from build123d import *

# Parameters (mm, degrees)
F3_DEPTH = 6
F4_R     = 4.8870891215
F5_DEPTH = 4.0010006557


with BuildPart() as f1:
    # F0 (on Front) → F1 (revolve)
    with BuildSketch(Plane.XZ):
        Polygon((-7.3680463247, -9.7499769181), (-20, -9.7499769181), (-20, -13.7499775738), (0, -13.7499775738), (0, 13.7500224262), (-4, 13.4215392172), (-4, -0.5182113382), (-7.3680463247, -0.5182113382), align=None)
    revolve(axis=Axis((0, 0, 2.24262e-05), (0, 0, 1)))

    # F2 (on face) → F3 (join)
    with BuildSketch(Plane.XY.offset(-0.5182113382)):
        Polygon((-1.4578928646, 3.7248554865), (1.4578928646, 3.7248554865), (0, 6.25), align=None)
        Polygon((-3.954765909, -0.5998554865), (-5.4126587737, -3.125), (-2.4968730444, -3.125), align=None)
        Polygon((2.4968730444, -3.125), (5.4126587737, -3.125), (3.954765909, -0.5998554865), align=None)
    extrude(amount=F3_DEPTH)

    # F4 (on face) → F5 (cut, through all)
    with BuildSketch(Plane.XY.offset(-9.7499769181)):
        with Locations((12.3, 0)):
            Circle(F4_R)
    extrude(amount=-F5_DEPTH, mode=Mode.SUBTRACT)


solid = f1.part
Geometry check sheet. Reference: the model listing, model coordinates, mm. A direction names the side the tool comes from. Round coordinates to 2 decimals unless told otherwise and drop trailing zeros. Loops run counter-clockwise (first coordinate to the right, second up) from the corner with the lowest first, then second, coordinate; pieces in that order, holes last.
Item 1: Gauge pin test, flat ends, axial feed: pin 1 (0.8 mm diameter, centred on x = -0.5, y = 5.5, fed in from +Z); pin 2 (12.5 mm diameter, centred on x = 12.3, y = 0, fed in from +Z); pin 3 (2 mm diameter, centred on y = -2, z = 3, fed in from -X); pin 4 (10 mm diameter, centred on x = 15.5, z = 4, fed in from +Y). Record the tip position at first contact, or that the pin passes through.
Item 2: Access from +Z, -Z, +X, -X, +Y, -Y to the whole of each face (thin tool, end or side, straight path). Record for faces 4 (the flat face through (-0.719, 5.005, 2.44)), 5 (the cylindrical face through (-3.4, 6.537, -5.199)), 6 (the flat face through (4, -2, 5.482)).
Item 3: Cross-section at D-D on z = 11.25. Record the boundary of the cut face in (x, y).
Item 4: Cross-section at B-B on x = 12.3. Record the boundary of the cut face in (y, z).
Item 5: Thickness scan on line 1 (Z direction, x = -6, y = -14.5); line 2 (Y direction, x = 12.3, z = -11.15); line 3 (X direction, y = 4, z = -10.75). Record the ranges inside material, lowest first.
Item 6: Cross-section at C-C on y = -12. Record the boundary of the cut face in (x, z), then the cut area to 3 significant figures.
Item 7: Mould release check, pull along X, two halves, no side actions. Record for faces 1 (the cylindrical face through (0.867, 3.905, 6.354)), 2 (the flat face through (-4, -3.125, 2)), 3 (the cylindrical face through (8.42, -2.97, -11.72)): pulls with the +X half, pulls with the -X half, needs draft (parallel to the pull), parting line crosses it, or undercut.
Item 8: Cross-section at A-A on z = 2.5. Record the boundary of the cut face in (x, y) (3 decimals), then the cut area to 3 significant figures.
Answer sheet:
1. pin 1: stops at z = 5.48
1. pin 2: stops at z = -0.52
1. pin 3: stops at x = -5.34
1. pin 4: passes through
2. face 4: +Z, -X, +Y
2. face 5: +Z
2. face 6: +Z, +X, -Y
3. outline: circle Ø8 at (0, 0)
4. outline: (-15.77, -13.75) - (-4.89, -13.75) - (-4.89, -9.75) - (-15.77, -9.75) - close; (4.89, -13.75) - (15.77, -13.75) - (15.77, -9.75) - (4.89, -9.75) - close
5. line 1: z = -13.75 to -9.75
5. line 2: y = -15.77 to -4.89, 4.89 to 15.77
5. line 3: x = -19.6 to 9.49, 15.11 to 19.6
6. outline: (-16, -13.75) - (16, -13.75) - (16, -9.75) - (-16, -9.75) - close
6. area: 128 mm2
7. face 1: parting line crosses it
7. face 2: needs draft
7. face 3: undercut
8. outline: (-5.413, -3.125) - (-2.497, -3.125) arc R4 ccw to (2.497, -3.125) - (5.413, -3.125) - (3.955, -0.6) arc R4 ccw to (1.458, 3.725) - (0, 6.25) - (-1.458, 3.725) arc R4 ccw to (-3.955, -0.6) - close
8. area: 59.7 mm2
